```python
from build123d import *

# Parameters (mm, degrees)
SKETCH2_W           = 108
SKETCH2_H           = 72
BOSS_EXTRUDE1_DEPTH = 20.64
SHELL1_T            = 5
SKETCH3_W           = 118
SKETCH3_H           = 82
CUT_EXTRUDE1_DEPTH  = 3
SKETCH4_W           = 15
SKETCH4_H           = 15
SKETCH4_R           = 3.3
BOSS_EXTRUDE2_DEPTH = 3.175
FILLET1_R           = 10
FILLET2_R           = 8
CUT_EXTRUDE2_DEPTH  = 1.875


with BuildPart() as part:
    # Sketch2 → Boss-Extrude1 (new body)
    with BuildSketch(Plane.XY):
        Rectangle(SKETCH2_W, SKETCH2_H)
    extrude(amount=BOSS_EXTRUDE1_DEPTH)

    # Shell1
    shell1_openings = [part.faces().sort_by_distance(p)[0] for p in [
        (0, 0, 20.64),
    ]]
    offset(amount=SHELL1_T, openings=shell1_openings, kind=Kind.INTERSECTION)

    # Sketch3 → Cut-Extrude1 (cut)
    with BuildSketch(Plane(origin=(0, 0, -5), x_dir=(-1, 0, 0), z_dir=(0, 0, -1))):
        Rectangle(SKETCH3_W, SKETCH3_H)
    extrude(amount=-CUT_EXTRUDE1_DEPTH, mode=Mode.SUBTRACT)

    # Sketch4 → Boss-Extrude2 (add)
    # profile 1 of 2: a face of its own
    with BuildSketch(Plane.XZ.offset(41)):
        with Locations((-66.5, 9.32)):
            Rectangle(SKETCH4_W, SKETCH4_H)
        with Locations(Location((-66.5, 9.32, 0), (0, 0, 270))):
            Circle(SKETCH4_R, mode=Mode.SUBTRACT)
    # profile 2 of 2: a face of its own
    with BuildSketch(Plane.XZ.offset(41)):
        with Locations((66.5, 9.32)):
            Rectangle(SKETCH4_W, SKETCH4_H)
        with Locations(Location((66.5, 9.32, 0), (0, 0, 270))):
            Circle(SKETCH4_R, mode=Mode.SUBTRACT)
    extrude(amount=-BOSS_EXTRUDE2_DEPTH)

    # Fillet1
    fillet1_edges = [part.edges().sort_by_distance(p)[0] for p in [
        (54, -36, 10.32),
        (54, 36, 10.32),
        (-54, 36, 10.32),
        (-54, -36, 10.32),
        (-59, 41, 9.32),
        (59, 41, 9.32),
    ]]
    fillet(fillet1_edges, radius=FILLET1_R)

    # Fillet2
    # the kernel refuses this fillet: 8 mm, written as the material it adds along each edge
    with BuildSketch(Plane(origin=(59, -41, 16.82), x_dir=(0, 0, 1), z_dir=(0, 1, 0)), Plane(origin=(-59, -41, 1.82), x_dir=(0, 0, -1), z_dir=(0, 1, 0))) as fillet2_piece_1:
        with BuildLine():
            CenterArc((8, 6.821114278), FILLET2_R, 180, 58.499903552)
            Line((0, 6.821114278), (0, 0))
            Line((0, 0), (3.82, 0))
        make_face()
    extrude(amount=3.175)
    with BuildSketch(Plane(origin=(59, -41, 1.82), x_dir=(0, 0, -1), z_dir=(0, 1, 0)), Plane(origin=(-59, -41, 16.82), x_dir=(0, 0, 1), z_dir=(0, 1, 0))) as fillet2_piece_2:
        with BuildLine():
            CenterArc((8, -6.821114278), FILLET2_R, 121.500096448, 58.499903552)
            Line((0, -6.821114278), (0, 0))
            Line((0, 0), (3.82, 0))
        make_face()
    extrude(amount=3.175)
    # the kernel refuses this fillet: 8 mm, written as the material it takes off along each edge
    with BuildSketch(Plane(origin=(74, -61, 16.82), x_dir=(0, 0, -1), z_dir=(0, 1, 0)), Plane(origin=(-74, -61, 1.82), x_dir=(0, 0, 1), z_dir=(0, 1, 0)), Plane(origin=(-74, -61, 16.82), x_dir=(1, 0, 0), z_dir=(0, 1, 0))) as fillet2_2_piece_1:
        with BuildLine():
            CenterArc((FILLET2_R, FILLET2_R), FILLET2_R, 180, 90)
            Line((0, FILLET2_R), (0, 0))
            Line((0, 0), (FILLET2_R, 0))
        make_face()
    extrude(amount=43.175, mode=Mode.SUBTRACT)
    with BuildSketch(Plane(origin=(74, -61, 1.82), x_dir=(0, 0, 1), z_dir=(0, 1, 0))) as fillet2_2_piece_2:
        with BuildLine():
            CenterArc((FILLET2_R, -FILLET2_R), FILLET2_R, 90, 90)
            Line((0, -FILLET2_R), (0, 0))
            Line((0, 0), (FILLET2_R, 0))
        make_face()
    extrude(amount=43.175, mode=Mode.SUBTRACT)

    # Sketch5 → Cut-Extrude2 (cut)
    with BuildSketch(Plane.XY.offset(20.64)):
        with BuildLine():
            Line((46.071067812, -39.11), (-46.071067812, -39.11))
            ThreePointArc((-46.071067812, -39.11), (-54.050767838, -35.804700026), (-57.356067812, -27.825))
            Line((-57.356067812, -27.825), (-57.356067812, 28.071067812))
            ThreePointArc((-57.356067812, 28.071067812), (-54.050767838, 36.050767838), (-46.071067812, 39.356067812))
            Line((-46.071067812, 39.356067812), (46.071067812, 39.356067812))
            ThreePointArc((46.071067812, 39.356067812), (54.050767838, 36.050767838), (57.356067812, 28.071067812))
            Line((57.356067812, 28.071067812), (57.356067812, -27.825))
            ThreePointArc((57.356067812, -27.825), (54.050767838, -35.804700026), (46.071067812, -39.11))
        make_face()
        with BuildLine():
            Line((46.071067812, -36.54), (-46.071067812, -36.54))
            ThreePointArc((-46.071067812, -36.54), (-52.23350341, -33.987435598), (-54.786067812, -27.825))
            Line((-54.786067812, -27.825), (-54.786067812, 28.071067812))
            ThreePointArc((-54.786067812, 28.071067812), (-52.23350341, 34.23350341), (-46.071067812, 36.786067812))
            Line((-46.071067812, 36.786067812), (46.071067812, 36.786067812))
            ThreePointArc((46.071067812, 36.786067812), (52.23350341, 34.23350341), (54.786067812, 28.071067812))
            Line((54.786067812, 28.071067812), (54.786067812, -27.825))
            ThreePointArc((54.786067812, -27.825), (52.23350341, -33.987435598), (46.071067812, -36.54))
        make_face(mode=Mode.SUBTRACT)
    extrude(amount=-CUT_EXTRUDE2_DEPTH, mode=Mode.SUBTRACT)


solid = part.part
```
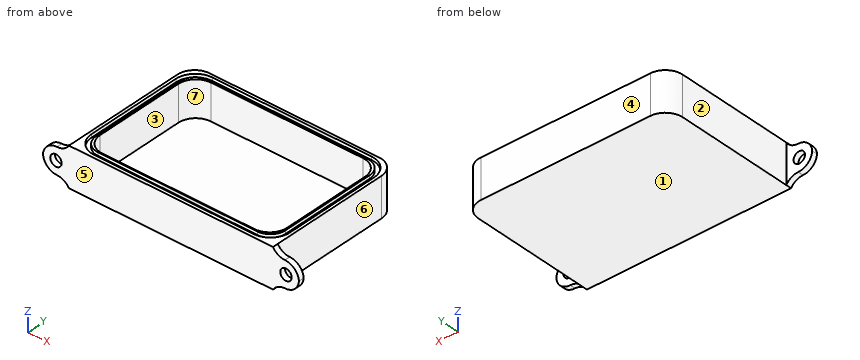
Could you check a few things on this model? Use its own coordinates, in mm. Face numbers are marked on the shaded views. A direction names the side the tool comes from. Coordinates: 2 decimals unless noted, no trailing zeros. Write each loop counter-clockwise with the first axis right and the second up, starting at its lowest first coordinate (ties: lowest second). Pieces come first, ordered by that corner, then holes. Notation, with made-up numbers: (39, 77) -> (83, 77) arc R19 ccw to (83, 84) -> close; hole circle Ø7 at (65.5, 72.25). An arc over 180 degrees is marked (long way). One line per question, with ' | ' between items. Start each with the question number.
1. Will these pins go through, and if not, where does the flat tip stop? P1, Ø6, axis at y = -15.5, z = 15.5, coming from the -X side; P2, Ø10.5, axis at y = -7, z = 13, coming from the +X side; P3, Ø5.5, axis at x = -66.5, z = 9.32, coming from the +Y side; P4, Ø1, axis at x = 13.5, y = -18.5, coming from the +Z side.
2. If we section it at B-B (y = 11.5): Please give me the cut outline in (x, z) (3 decimals), and give its area (3 significant figures).
3. If we section it at A-A (z = 7.5): Please give me the cut outline in (x, y) (3 decimals), and give its area (3 significant figures).
4. Thinking about a two-plate mould opening in Y: for the marked faces 4, 5, 6 and 7, which applies, pulls with the +Y half, pulls with the -Y half, needs draft (parallel to the pull), parting line crosses it, or undercut?
5. If we section it at C-C (z = 15): Please give me the cut outline in (x, y) (3 decimals).
6. For the marked faces 1, 2 and 3, which set-ups out of +Z, -Z, +X, -X, +Y, -Y let a thin tool reach every point of the face, with its end or its side?
7. Please list where these lines run through material, in increasing order: line 1 along X through (y, z) = (-40.1, 9.32); line 2 along Y through (x, z) = (-3, 19.75); line 3 along Y through (x, z) = (-16, 18.5).
8. If we section it at D-D (y = 34): Please give me the cut outline in (x, z) (3 decimals), and give its area (3 significant figures).
Return value:
1) P1: stops at x = -59 | P2: stops at x = 59 | P3: passes through | P4: stops at z = 0
2) outline: (-59, -2) -> (59, -2) -> (59, 20.64) -> (57.356, 20.64) -> (57.356, 18.765) -> (54.786, 18.765) -> (54.786, 20.64) -> (54, 20.64) -> (54, 0) -> (-54, 0) -> (-54, 20.64) -> (-54.786, 20.64) -> (-54.786, 18.765) -> (-57.356, 18.765) -> (-57.356, 20.64) -> (-59, 20.64) -> close | area: 433 mm²
3) outline: (-73.656, -41) -> (-69.253, -41) -> (-69.253, -37.825) -> (-73.656, -37.825) -> close; (-63.747, -41) -> (63.747, -41) -> (63.747, -37.825) -> (59, -37.825) -> (59, 31) arc R10 ccw to (49, 41) -> (-49, 41) arc R10 ccw to (-59, 31) -> (-59, -37.825) -> (-63.747, -37.825) -> close; (69.253, -41) -> (73.656, -41) -> (73.656, -37.825) -> (69.253, -37.825) -> close; hole (-54, -26) arc R10 ccw to (-44, -36) -> (44, -36) arc R10 ccw to (54, -26) -> (54, 26) arc R10 ccw to (44, 36) -> (-44, 36) arc R10 ccw to (-54, 26) -> close | area: 2,000 mm²
4) face 4: pulls with the +Y half | face 5: pulls with the -Y half | face 6: needs draft | face 7: undercut
5) outline: (-71.08, -41) -> (71.08, -41) -> (71.08, -37.825) -> (59, -37.825) -> (59, 31) arc R10 ccw to (49, 41) -> (-49, 41) arc R10 ccw to (-59, 31) -> (-59, -37.825) -> (-71.08, -37.825) -> close; hole (-54, -26) arc R10 ccw to (-44, -36) -> (44, -36) arc R10 ccw to (54, -26) -> (54, 26) arc R10 ccw to (44, 36) -> (-44, 36) arc R10 ccw to (-54, 26) -> close
6) face 1: -Z, +X, -X, +Y, -Y | face 2: +Z, -Z, -X, +Y | face 3: +Z
7) line 1: x = -73.98 to -69.8, -63.2 to 63.2, 69.8 to 73.98 | line 2: y = -41 to -39.11, -36.54 to -36, 36 to 36.79, 39.36 to 41 | line 3: y = -41 to -36, 36 to 41
8) outline: (-58.539, -2) -> (58.539, -2) -> (58.539, 20.64) -> (55.673, 20.64) -> (55.673, 18.765) -> (52.458, 18.765) -> (52.458, 20.64) -> (50, 20.64) -> (50, 0) -> (-50, 0) -> (-50, 20.64) -> (-52.458, 20.64) -> (-52.458, 18.765) -> (-55.673, 18.765) -> (-55.673, 20.64) -> (-58.539, 20.64) -> close | area: 575 mm²
